Could you check a few things on this model? Use its own coordinates, in mm. Face numbers are marked on the shaded views. A direction names the side the tool comes from. Coordinates: 2 decimals unless noted, no trailing zeros. Order: outer loops, then holes, each group sorted by start corner. A loop starts at its lowest first (then second) coordinate and runs counter-clockwise, first axis right, second up. Notation, with made-up numbers: (88, 42.25) - (119, 42.25) arc R13 ccw to (119, 49.25) - close; hole circle Ø1 at (16.25, 70). An arc over 180 degrees is marked (long way). One line per item, written item: value.
from build123d import *

# Parameters (mm, degrees)
F0_W     = 43.2214178145
F0_H     = 13.4684350342
F2_R     = 19.05
F3_DEPTH = 152.4
F4_R     = 5.08
F5_DEPTH = 5.08
F6_R     = 2.3709627479
F7_DEPTH = 25.4
F8_SIZE  = 2.54
F9_R     = 5.08
F10_D    = 6.6


with BuildPart() as f1:
    # F0 (on Front) → F1 (revolve)
    with BuildSketch(Plane.XZ):
        with Locations((21.6107089072, 6.7342175171)):
            Rectangle(F0_W, F0_H)
    revolve(axis=Axis((0, 0, 6.7342175171), (0, 0, 1)))

    # F2 (on face) → F3 (join)
    with BuildSketch(Plane(origin=(0, 0, 0), x_dir=(1, 0, 0), z_dir=(0, 0, -1))):
        Circle(F2_R)
    extrude(amount=-F3_DEPTH)

    # F4 (on face) → F5 (cut)
    with BuildSketch(Plane.XY.offset(13.4684350342)):
        with Locations((-24.6729586924, 21.0248965081)):
            Circle(F4_R)
        with Locations((24.8374585062, 21.8454711139)):
            Circle(F4_R)
        with Locations((-25.066871196, -20.6134561449)):
            Circle(F4_R)
        with Locations((24.5745163411, -20.6259563565)):
            Circle(F4_R)
    extrude(amount=-F5_DEPTH, mode=Mode.SUBTRACT)

    # F6 (on face) → F7 (cut)
    with BuildSketch(Plane.XY.offset(13.4684350342)):
        with Locations((-25.066871196, -20.6134561449)):
            Circle(F6_R)
        with Locations((24.4725923985, -20.7640305161)):
            Circle(F6_R)
        with Locations((24.4725923985, 21.6897111386)):
            Circle(F6_R)
        with Locations((-24.7867107391, 21.3656388223)):
            Circle(F6_R)
    extrude(amount=-F7_DEPTH, mode=Mode.SUBTRACT)

    # F8
    f8_edges = [f1.edges().sort_by_distance(p)[0] for p in [
        (-19.05, 0, 152.4),
        (-43.221418, 0, 13.468435),
    ]]
    chamfer(f8_edges, length=F8_SIZE)

    # F9
    f9_edges = [f1.edges().sort_by_distance(p)[0] for p in [
        (-19.05, 0, 13.468435),
    ]]
    fillet(f9_edges, radius=F9_R)

    # F10 (through all)
    with Locations(Plane.XY.offset(13.4684350342)):
        with Locations((24.4725923985, -20.7640305161)):
            Hole(F10_D / 2)


solid = f1.part
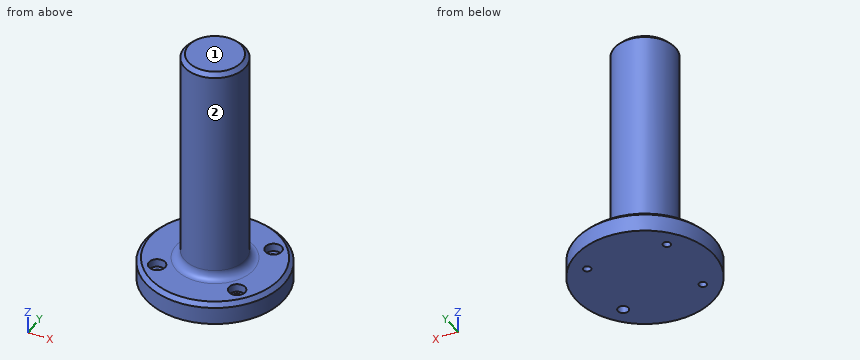
Item 1: I want a section at C-C on z = 76.5. Please give me the cut outline in (x, y), then the cut area to 3 significant figures.
Conclusion:
outline: circle Ø38.1 at (0, 0)
area: 1,140 mm²
Item 2: I'm going to push flat-ended pins straight in: pin 1 Ø2 at (x, y) = (-21.5, -12.5) entering from +Z; pin 2 Ø5.5 at (x, y) = (24.47, -20.76) entering from -Z; pin 3 Ø2 at (x, z) = (-7.5, 18) entering from -Y; pin 4 Ø5 at (x, y) = (24, -22.5) entering from +Z. Where does each tip first touch, or does it pass through?
Conclusion:
pin 1: z = 13.48
pin 2: through
pin 3: y = -17.97
pin 4: z = 8.39
Item 3: I want a section at A-A on x = 0. Please give me the cut outline in (y, z), then the cut area to 3 significant figures.
Conclusion:
outline: (-43.22, 0) - (43.22, 0) - (43.22, 10.93) - (40.68, 13.47) - (24.13, 13.47) arc R5.08 cw to (19.05, 18.55) - (19.05, 149.86) - (16.51, 152.4) - (-16.51, 152.4) - (-19.05, 149.86) - (-19.05, 18.55) arc R5.08 cw to (-24.13, 13.47) - (-40.68, 13.47) - (-43.22, 10.93) - close
area: 6,460 mm²
Item 4: For the marked faces 1 and 2, which set-ups out of +Z, -Z, +X, -X, +Y, -Y let a thin tool reach every point of the face, with its end or its side?
Conclusion:
face 1: +Z, +X, -X, +Y, -Y
face 2: +Z
Item 5: If I drill on probe 1 along Z at (x, y) = (25.5, -17.5); probe 2 along Z at (x, y) = (16.5, -34); probe 3 along X at (y, z) = (9.5, 118), over which ranges is the centre line in solid material (lowest first)?
Conclusion:
probe 1: 0 to 8.39
probe 2: 0 to 13.47
probe 3: -16.51 to 16.51
